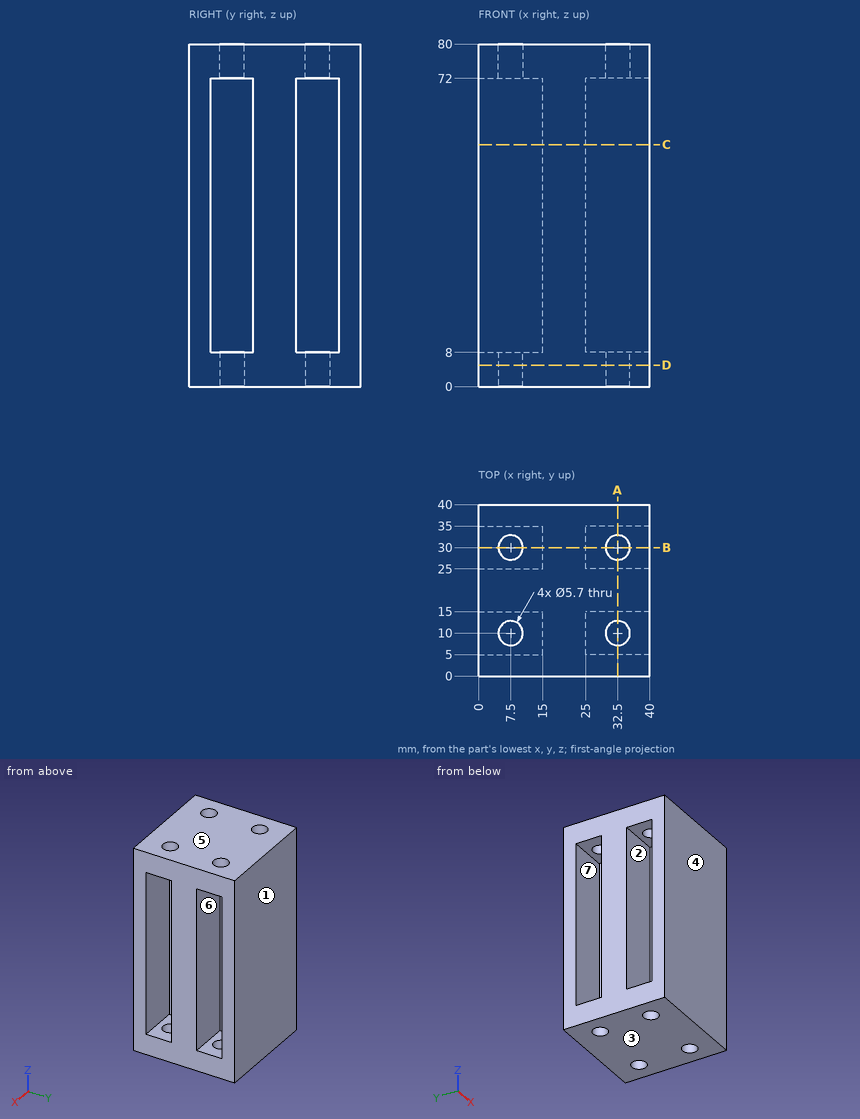
Input: dimensioned drawing with shaded views. Units: mm. Origin: part minimum x, y, z. A direction names the side the tool comes from. Coordinates: 2 decimals unless noted, no trailing zeros. Order: outer loops, then holes, each group sorted by start corner. A loop starts at its lowest first (then second) coordinate and runs counter-clockwise, first axis right, second up.
(1) First-contact query: pin 1 (2 mm diameter, centred on y = 27, z = 26.5, fed in from +X); pin 2 (5 mm diameter, centred on y = 8, z = 52.5, fed in from -X). Flat tips, straight axial feed; report the tip coordinate or a pass-through.
(2) Section query D-D (z = 5). Return the cut outline in (x, y), plus the area to 3 significant figures.
(3) Material intervals for probe 1 along Y at (x, z) = (29.5, 69.5); probe 2 along Y at (x, z) = (32.5, 78); probe 3 along Z at (x, y) = (6, 14), sorted ascending.
(4) Section query C-C (z = 56.5). Return the cut outline in (x, y).
(5) Section query A-A (x = 32.5). Return the cut outline in (y, z).
(6) Draft query along Y for the marked faces 1, 2, 3 and 4. Return one class per face: pulls with the +Y half, pulls with the -Y half, needs draft (parallel to the pull), parting line crosses it, or undercut.
(7) Access query for the marked faces 5, 6 and 7. Directions: +Z, -Z, +X, -X, +Y, -Y. A direction counts if a zero-diameter tool reaches every point of the face in a straight line with its end or side. Return the directions, or none.
(8) Section query B-B (y = 30). Return the cut outline in (x, z), plus the area to 3 significant figures.
Solution:
1. pin 1: stops at x = 25
1. pin 2: stops at x = 15
2. outline: (0, 0) - (40, 0) - (40, 40) - (0, 40) - close; hole circle Ø5.7 at (7.5, 10); hole circle Ø5.7 at (7.5, 30); hole circle Ø5.7 at (32.5, 10); hole circle Ø5.7 at (32.5, 30)
2. area: 1,500 mm2
3. probe 1: y = 0 to 5, 15 to 25, 35 to 40
3. probe 2: y = 0 to 7.15, 12.85 to 27.15, 32.85 to 40
3. probe 3: z = 0 to 8, 72 to 80
4. outline: (0, 0) - (40, 0) - (40, 5) - (25, 5) - (25, 15) - (40, 15) - (40, 25) - (25, 25) - (25, 35) - (40, 35) - (40, 40) - (0, 40) - (0, 35) - (15, 35) - (15, 25) - (0, 25) - (0, 15) - (15, 15) - (15, 5) - (0, 5) - close
5. outline: (0, 0) - (7.15, 0) - (7.15, 8) - (5, 8) - (5, 72) - (7.15, 72) - (7.15, 80) - (0, 80) - close; (12.85, 0) - (27.15, 0) - (27.15, 8) - (25, 8) - (25, 72) - (27.15, 72) - (27.15, 80) - (12.85, 80) - (12.85, 72) - (15, 72) - (15, 8) - (12.85, 8) - close; (32.85, 0) - (40, 0) - (40, 80) - (32.85, 80) - (32.85, 72) - (35, 72) - (35, 8) - (32.85, 8) - close
6. face 1: pulls with the +Y half
6. face 2: undercut
6. face 3: needs draft
6. face 4: pulls with the -Y half
7. face 5: +Z, +X, -X, +Y, -Y
7. face 6: +X
7. face 7: -X
8. outline: (0, 0) - (4.65, 0) - (4.65, 8) - (0, 8) - close; (0, 72) - (4.65, 72) - (4.65, 80) - (0, 80) - close; (10.35, 0) - (29.65, 0) - (29.65, 8) - (25, 8) - (25, 72) - (29.65, 72) - (29.65, 80) - (10.35, 80) - (10.35, 72) - (15, 72) - (15, 8) - (10.35, 8) - close; (35.35, 0) - (40, 0) - (40, 8) - (35.35, 8) - close; (35.35, 72) - (40, 72) - (40, 80) - (35.35, 80) - close
8. area: 1,100 mm2
